The model under review builds one solid part; all positions refer to its coordinate system, in mm. Face numbers are marked on the shaded views. A direction names the side the tool comes from. Give positions to 0.01 mm unless a question says otherwise; leave off trailing zeros. Order: outer loops, then holes, each group sorted by start corner. A loop starts at its lowest first (then second) coordinate and runs counter-clockwise, first axis right, second up.
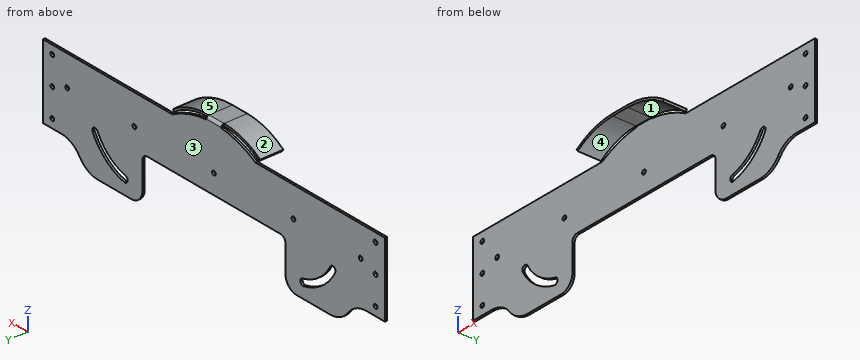
```python
from build123d import *

# Parameters (mm, degrees)
SKETCH1_W          = 584.2
SKETCH1_H          = 304.8
BASE_FLANGE1_DEPTH = 3.175
SKETCH6_R          = 3.175
CUT_EXTRUDE1_DEPTH = 340.318162239
CUT_EXTRUDE2_DEPTH = 340.318162239
EDGE_FLANGE1_DEPTH = 25.4
HEM1_START         = -38.1
HEM1_DEPTH         = 34.1884
FILLET1_R          = 1.5875
SKETCH16_R         = 3.175
CUT_EXTRUDE3_DEPTH = 328.883956385
CUT_EXTRUDE4_DEPTH = 328.883956385
FILLET3_R          = 19.05


# Read off the part's stored shape, not the designer's step: Hem1
# Sheet-metal steps are written as plain solids
with BuildPart() as part:
    # Sketch1 → Base-Flange1 (new body)
    with BuildSketch(Plane(origin=(0, 0, 0), x_dir=(1, 0, 0), z_dir=(0, 1, 0))):
        with Locations((0, -20.239290429)):
            Rectangle(SKETCH1_W, SKETCH1_H)
    extrude(amount=-BASE_FLANGE1_DEPTH)

    # Sketch6 → Cut-Extrude1 (cut, through all)
    with BuildSketch(Plane(origin=(0, 0, 0), x_dir=(1, 0, 0), z_dir=(0, 1, 0))):
        with Locations(Location((-135.858839885, -76.581, 0), (0, 0, 270))):
            Circle(SKETCH6_R)
        with Locations(Location((135.858839885, -76.581, 0), (0, 0, 90))):
            Circle(SKETCH6_R)
        with BuildLine():
            ThreePointArc((-153.343024391, 2.471069539), (-184.826505048, -12.105468402), (-207.318024391, -38.521686343))
            ThreePointArc((-207.318024391, -38.521686343), (-205.353326106, -44.963950941), (-198.911061508, -42.999252655))
            ThreePointArc((-198.911061508, -42.999252655), (-179.065603264, -19.690825061), (-151.286061508, -6.829173936))
            ThreePointArc((-151.286061508, -6.829173936), (-147.664421212, -1.150570757), (-153.343024391, 2.471069539))
        make_face()
        with BuildLine():
            ThreePointArc((153.343024391, 2.471069539), (184.826505048, -12.105468402), (207.318024391, -38.521686343))
            ThreePointArc((207.318024391, -38.521686343), (205.353326106, -44.963950941), (198.911061508, -42.999252655))
            ThreePointArc((198.911061508, -42.999252655), (179.065603264, -19.690825061), (151.286061508, -6.829173936))
            ThreePointArc((151.286061508, -6.829173936), (147.664421212, -1.150570757), (153.343024391, 2.471069539))
        make_face()
    extrude(amount=-CUT_EXTRUDE1_DEPTH, mode=Mode.SUBTRACT)

    # Sketch7 → Cut-Extrude2 (cut, through all)
    with BuildSketch(Plane(origin=(0, 0, 0), x_dir=(1, 0, 0), z_dir=(0, 1, 0))):
        with BuildLine():
            Line((292.1, -120.65), (260.35, -120.65))
            Line((260.35, -120.65), (71.177693563, -120.65))
            ThreePointArc((71.177693563, -120.65), (42.985302493, -133.322729985), (12.7, -139.504109477))
            Line((12.7, -139.504109477), (12.7, -140.081))
            Line((12.7, -140.081), (-12.7, -140.081))
            Line((-12.7, -140.081), (-12.7, -139.504109477))
            ThreePointArc((-12.7, -139.504109477), (-42.985302493, -133.322729985), (-71.177693563, -120.65))
            Line((-71.177693563, -120.65), (-260.35, -120.65))
            Line((-260.35, -120.65), (-292.1, -120.65))
            Line((-292.1, -120.65), (-292.1, -172.639290429))
            Line((-292.1, -172.639290429), (292.1, -172.639290429))
            Line((292.1, -172.639290429), (292.1, -120.65))
        make_face()
        with BuildLine():
            Line((260.35, -12.7), (292.1, -12.7))
            Line((292.1, -12.7), (292.1, 132.160709571))
            Line((292.1, 132.160709571), (-292.1, 132.160709571))
            Line((-292.1, 132.160709571), (-292.1, -12.7))
            Line((-292.1, -12.7), (-260.35, -12.7))
            ThreePointArc((-260.35, -12.7), (-242.959808799, -8.49972345), (-229.403927955, 3.175))
            ThreePointArc((-229.403927955, 3.175), (-215.848047111, 14.84972345), (-198.45785591, 19.05))
            Line((-198.45785591, 19.05), (198.45785591, 19.05))
            ThreePointArc((198.45785591, 19.05), (215.848047111, 14.84972345), (229.403927955, 3.175))
            ThreePointArc((229.403927955, 3.175), (242.959808799, -8.49972345), (260.35, -12.7))
        make_face()
    extrude(amount=-CUT_EXTRUDE2_DEPTH, mode=Mode.SUBTRACT)

    # Edge-Flange1 section (across the edge) → Edge-Flange1 (add)
    with BuildSketch(Plane(origin=(12.7, -3.175, 140.8176), x_dir=(0, 0, -1), z_dir=(-1, 0, 0))):
        with BuildLine():
            Line((-3.175, 0.7366), (-3.175, 34.925))
            Line((-3.175, 34.925), (0, 34.925))
            Line((0, 34.925), (0, 0.7366))
            ThreePointArc((0, 0.7366), (0.215745145, 0.215745145), (0.7366, 0))
            Line((0.7366, 0), (0.7366, -3.175))
            ThreePointArc((0.7366, -3.175), (-2.029318885, -2.029318885), (-3.175, 0.7366))
        make_face()
    extrude(amount=EDGE_FLANGE1_DEPTH)

    # Hem1 outline → Hem1 (add)
    with BuildSketch(Plane(origin=(0, 0, 0), x_dir=(1, 0, 0), z_dir=(0, 1, 0)).offset(HEM1_START)):
        with BuildLine():
            Line((-72.650782704, -121.915190821), (-74.471887889, -124.515998562))
            ThreePointArc((-74.471887889, -124.515998562), (-45.084811783, -139.008100728), (-12.7, -143.9926))
            Line((-12.7, -143.9926), (-12.7, -140.8176))
            ThreePointArc((-12.7, -140.8176), (-44.13007087, -135.980049409), (-72.650782704, -121.915190821))
        make_face()
        with BuildLine():
            Line((74.471887889, -124.515998562), (72.650782704, -121.915190821))
            ThreePointArc((72.650782704, -121.915190821), (44.13007087, -135.980049409), (12.7, -140.8176))
            Line((12.7, -140.8176), (12.7, -143.9926))
            ThreePointArc((12.7, -143.9926), (45.084811783, -139.008100728), (74.471887889, -124.515998562))
        make_face()
    extrude(amount=HEM1_DEPTH)

    # Fillet1
    fillet1_edges = [part.edges().sort_by_distance(p)[0] for p in [
        (-71.177693563, -1.5875, 120.65),
        (71.177693563, -1.5875, 120.65),
    ]]
    fillet(fillet1_edges, radius=FILLET1_R)

    # Sketch16 → Cut-Extrude3 (cut, through all)
    with BuildSketch(Plane(origin=(0, 0, 0), x_dir=(1, 0, 0), z_dir=(0, 1, 0))):
        with Locations(Location((0, -76.2, 0), (0, 0, 270))):
            Circle(SKETCH16_R)
        with Locations(Location((-276.225, -25.4, 0), (0, 0, 270))):
            Circle(SKETCH16_R)
        with Locations(Location((-276.225, -107.95, 0), (0, 0, 270))):
            Circle(SKETCH16_R)
        with Locations(Location((-250.825, -76.2, 0), (0, 0, 270))):
            Circle(SKETCH16_R)
        with Locations(Location((276.225, -66.675, 0), (0, 0, 270))):
            Circle(SKETCH16_R)
        with Locations(Location((-276.225, -66.675, 0), (0, 0, 270))):
            Circle(SKETCH16_R)
        with Locations(Location((276.225, -107.95, 0), (0, 0, 270))):
            Circle(SKETCH16_R)
        with Locations(Location((276.225, -25.4, 0), (0, 0, 270))):
            Circle(SKETCH16_R)
        with Locations(Location((250.825, -76.2, 0), (0, 0, 270))):
            Circle(SKETCH16_R)
    extrude(amount=-CUT_EXTRUDE3_DEPTH, mode=Mode.SUBTRACT)

    # Sketch17 → Cut-Extrude4 (cut, through all)
    with BuildSketch(Plane(origin=(0, 0, 0), x_dir=(1, 0, 0), z_dir=(0, 1, 0))):
        with BuildLine():
            Line((-122.152042949, 19.05), (122.152042949, 19.05))
            Line((122.152042949, 19.05), (122.152042949, -39.6875))
            ThreePointArc((122.152042949, -39.6875), (119.827203025, -45.300160076), (114.214542949, -47.625))
            Line((114.214542949, -47.625), (-114.214542949, -47.625))
            ThreePointArc((-114.214542949, -47.625), (-119.827203025, -45.300160076), (-122.152042949, -39.6875))
            Line((-122.152042949, -39.6875), (-122.152042949, 19.05))
        make_face()
    extrude(amount=-CUT_EXTRUDE4_DEPTH, mode=Mode.SUBTRACT)

    # Fillet3
    fillet3_edges = [part.edges().sort_by_distance(p)[0] for p in [
        (122.152042949, -1.5875, -19.05),
        (-122.152042949, -1.5875, -19.05),
    ]]
    fillet(fillet3_edges, radius=FILLET3_R)


solid = part.part
```
Item 1: Clearance check with flat-ended pins moving along their axes: pin 1 Ø2.5 at (x, y) = (270.5, -1.5) entering from -Z; pin 2 Ø1 at (x, y) = (-47.5, -26) entering from +Z; pin 3 Ø1.5 at (y, z) = (-30, 123.5) entering from -X; pin 4 Ø6 at (x, z) = (137.5, 100.5) entering from +Y. State where each tip first meets the part, or that it passes through.
Values found:
pin 1: stops at z = 12.7
pin 2: stops at z = 138.38
pin 3: stops at x = -74.29
pin 4: stops at y = 0
Item 2: Take a section at A-A (x = 33). Give the boundary of the cut face in (y, z) (3 decimals), and give its area (3 significant figures).
Values found:
outline: (-38.1, 138.827) - (-3.912, 138.827) - (-3.912, 142.062) - (-38.1, 142.062) - close; (-3.175, 47.625) - (0, 47.625) - (0, 136.138) - (-3.175, 136.138) - close
area: 392 mm2
Item 3: For line 1 (X direction, y = -1.5, z = 76.2) (3 decimals); line 2 (Z direction, x = 2, y = -22); line 3 (X direction, y = -2, z = 20), list the stretches that pass through material, from the lowest coordinate up.
Values found:
line 1: x = -292.1 to -254, -247.65 to -139.011, -132.707 to -3.175, 3.175 to 132.707, 139.011 to 247.65, 254 to 292.1
line 2: z = 140.82 to 143.99
line 3: x = -292.1 to -193.77, -179.47 to -122.15, 122.15 to 179.47, 193.77 to 292.1
Item 4: Take a section at C-C (z = 130). Give the boundary of the cut face in (x, y) (3 decimals), and give its area (3 significant figures).
Values found:
outline: (-65.786, -38.1) - (-59.007, -38.1) - (-59.007, -3.912) - (-65.786, -3.912) - close; (-52.179, -3.175) - (52.179, -3.175) - (52.179, 0) - (-52.179, 0) - close; (59.007, -38.1) - (65.786, -38.1) - (65.786, -3.912) - (59.007, -3.912) - close
area: 795 mm2
Item 5: Take a section at B-B (y = -16). Give the boundary of the cut face in (x, z), and give its area (3 significant figures).
Values found:
outline: (-74.47, 124.52) - (-72.65, 121.92) arc R104.52 cw to (-12.7, 140.82) - (12.7, 140.82) arc R104.52 cw to (72.65, 121.92) - (74.47, 124.52) arc R107.7 ccw to (12.7, 143.99) - (-12.7, 143.99) arc R107.7 ccw to start
area: 492 mm2
Item 6: Draft analysis for pull direction X (two halves, no side actions). For the marked faces 3, 4 and 5, state which applies: released by +X, released by -X, zero draft, split by the parting line, or undercut.
Values found:
face 3: zero draft
face 4: undercut
face 5: released by +X
Item 7: For the marked faces 1 and 2, list the 3-axis set-ups (+Z, -Z, +X, -X, +Y, -Y) from which the entire face can be reached by the end or side of a thin tool; tool diameter is ignored.
Values found:
face 1: -Z, +Y, -Y
face 2: +Z, -X, +Y, -Y
